Can you work these out from the drawing? Everything is in mm from the part's minimum corner. A direction names the side the tool comes from. Round coordinates to 2 decimals unless told otherwise and drop trailing zeros. Loops run counter-clockwise (first coordinate to the right, second up) from the corner with the lowest first, then second, coordinate; pieces in that order, holes last. Notation, with made-up numbers: M 49.5,-12.5 L 91.5,-12.5 A13 ccw 91.5,12.5 Z; hole C -15.5,71.25 d1. An arc over 180 degrees is marked long. Use a Markdown table: item, result.
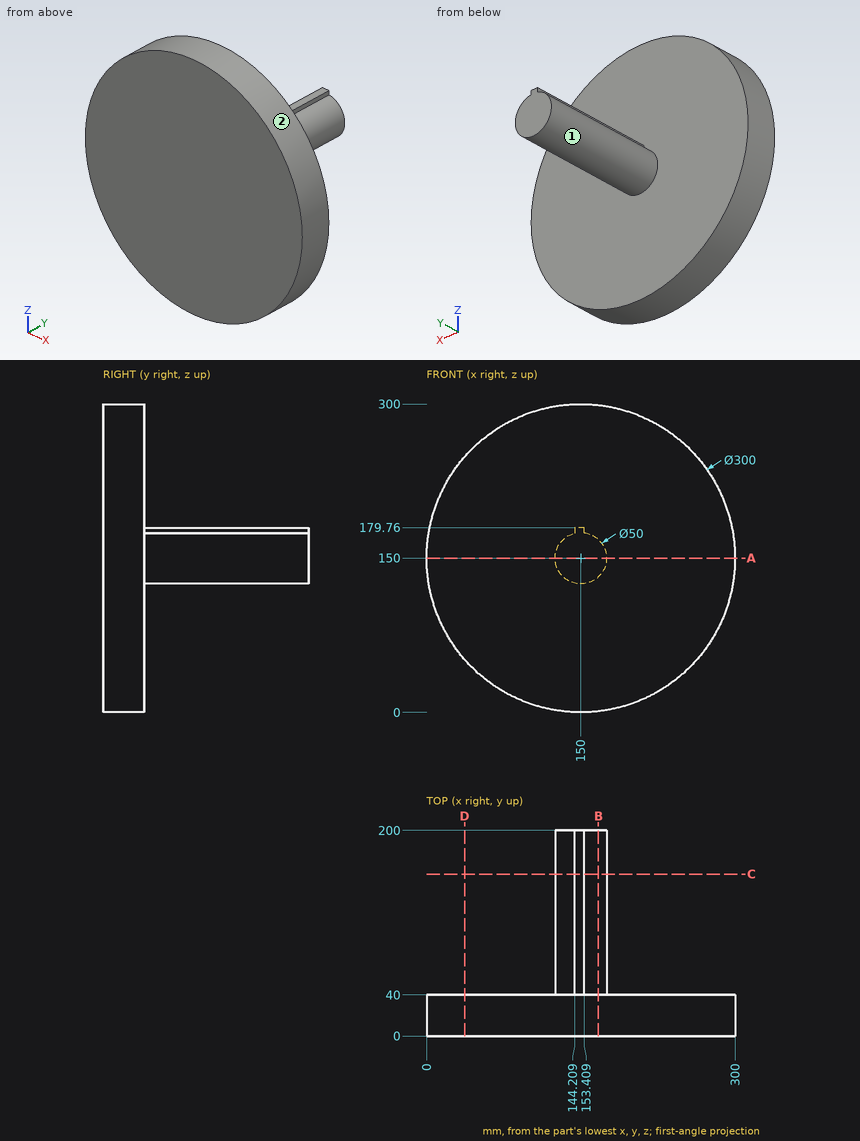
1. For pin 1 Ø6 at (x, z) = (84.5, 188.5) entering from +Y; pin 2 Ø8 at (x, y) = (240, 34.5) entering from +Z; pin 3 Ø10 at (x, y) = (150.5, 102.5) entering from +Z, each with a flat end and sliding along its axis, tell me the tip position at first contact or that it passes through.
Answer sheet:
| item | result |
|---|---|
| pin 1 | y = 40 |
| pin 2 | z = 272.9 |
| pin 3 | z = 179.76 |
2. Imagine slicing it at A-A, the plane z = 150. Write out the boundary of the cut face in (x, y).
Answer sheet:
| item | result |
|---|---|
| outline | M 0,0 L 300,0 L 300,40 L 175,40 L 175,200 L 125,200 L 125,40 L 0,40 Z |
3. Which directions (+Z, -Z, +X, -X, +Y, -Y) give clear straight access to the entire face, cutting with the end or side of a thin tool? Please do the marked faces 1 and 2.
Answer sheet:
| item | result |
|---|---|
| face 1 | +Y |
| face 2 | +Y, -Y |
4. Imagine slicing it at C-C, the plane y = 157.5. Write out the boundary of the cut face in (x, z).
Answer sheet:
| item | result |
|---|---|
| outline | M 144.21,174.32 A25 ccw long 153.41,174.77 L 153.41,179.76 L 144.21,179.76 Z |
5. I need wall thicknesses on probe 1 along Y at (x, z) = (202, 227); probe 2 along X at (y, z) = (48.5, 132); probe 3 along X at (y, z) = (77, 144.5). Which ranges of each line are inside material? Lowest first, please. Write a range as from..to.
Answer sheet:
| item | result |
|---|---|
| probe 1 | 0..40 |
| probe 2 | 132.65..167.35 |
| probe 3 | 125.61..174.39 |
6. Imagine slicing it at B-B, the plane x = 167. Write out the boundary of the cut face in (y, z).
Answer sheet:
| item | result |
|---|---|
| outline | M 0,0.97 L 40,0.97 L 40,131.67 L 200,131.67 L 200,168.33 L 40,168.33 L 40,299.03 L 0,299.03 Z |
7. Imagine slicing it at D-D, the plane x = 37. Write out the boundary of the cut face in (y, z).
Answer sheet:
| item | result |
|---|---|
| outline | M 0,51.35 L 40,51.35 L 40,248.65 L 0,248.65 Z |
